```python
from build123d import *

# Parameters (mm, degrees)
CUT_EXTRUDE1_DEPTH = 0.381
CIRPATTERN1_COUNT  = 2
CIRPATTERN1_ANGLE  = 90


with BuildPart() as part:
    # Sketch1 → Revolve1 (revolve)
    with BuildSketch(Plane.XY):
        with BuildLine():
            Line((2.794, 0.25), (2.794, 0))
            Line((2.794, 0), (1.13, 0))
            Line((1.13, 0), (1.13, -12.7))
            Line((1.13, -12.7), (0.125, -15.24))
            Line((0.125, -15.24), (0, -15.24))
            Line((0, -15.24), (0, 1.75))
            ThreePointArc((0, 1.75), (1.58559421, 1.351288149), (2.794, 0.25))
        make_face()
    revolve(axis=Axis((0, 0, 0), (0, 1, 0)))

    # Sketch2 → Cut-Extrude1 (cut, symmetric)
    with BuildSketch(Plane.XY):
        Polygon((-1.8, 2.20611304), (-0.381, 0.78711304), (0.381, 0.78711304), (1.8, 2.20611304), align=None)
    cut_extrude1 = extrude(amount=CUT_EXTRUDE1_DEPTH, both=True, mode=Mode.SUBTRACT)

    # CirPattern1: Cut-Extrude1 ×2 about axis
    cirpattern1_axis = Axis((0, 0, 0), (0, -1, 0))
    for i in range(1, CIRPATTERN1_COUNT):
        add(cut_extrude1.rotate(cirpattern1_axis, i * CIRPATTERN1_ANGLE / (CIRPATTERN1_COUNT - 1)), mode=Mode.SUBTRACT)


solid = part.part
```
Verification items for the finished model (mm, model axes). Coordinates: 2 decimals unless noted, no trailing zeros. Write each loop counter-clockwise with the first axis right and the second up, starting at its lowest first coordinate (ties: lowest second). Pieces come first, ordered by that corner, then holes. Notation, with made-up numbers: (3, 19.5) - (20, 19.5) arc R11 cw to (20, 23.5) - close; hole circle Ø11 at (15, 12.25). An arc over 180 degrees is marked (long way). Write item = value, one per line.
Q1. Cross-section at C-C (y = -13). Enter the section's corners in (x, z), plus the area to 3 significant figures.
Answer:
outline = circle Ø2.02 at (0, 0)
area = 3.21 mm²
Q2. Cross-section at A-A (y = -5.75). Enter the section's corners in (x, z).
Answer:
outline = circle Ø2.26 at (0, 0)
Q3. Cross-section at D-D (z = -2.25). Enter the section's corners in (x, y).
Answer:
outline = (-1.66, 0) - (1.66, 0) - (1.66, 0.25) arc R2.48 ccw to (-1.66, 0.25) - close
Q4. Go/stop test with flat-tipped pins: pin 1 Ø1 at (y, z) = (-10.5, -0.5) entering from +X; pin 2 Ø3 at (x, y) = (0.5, -4) entering from +Z; pin 3 Ø0.6 at (y, z) = (1.5, 0.5) entering from +X. Record where each tip stops, or that it passes through.
Answer:
pin_1 = 1.13
pin_2 = 1.13
pin_3 = 1.78
Q5. Cross-section at B-B (z = 1.9). Enter the section's corners in (x, y), plus the area to 3 significant figures.
Answer:
outline = (-2.05, 0) - (2.05, 0) - (2.05, 0.25) arc R2.76 ccw to (-2.05, 0.25) - close
area = 3.60 mm²
Q6. Material ranges on L1, parallel to Y at x = 1.9, z = -0.3; L2, parallel to X at y = -12.25, z = -0.9; L3, parallel to X at y = -8.5, z = 0.45, recorded low to high. Write a range as from..to.
Answer:
L1 = 0..1.14
L2 = -0.68..0.68
L3 = -1.04..1.04
